Here's the drawing with two shaded views (mm, measured from the low corner). I have some questions. Give positions to 0.01 mm unless a question says otherwise; leave off trailing zeros. Loops run counter-clockwise (first coordinate to the right, second up) from the corner with the lowest first, then second, coordinate; pieces in that order, holes last. Notation, with made-up numbers: (49, 29.25) - (60, 29.25) arc R21 ccw to (60, 53.25) - close; hole circle Ø4 at (-28, 0). An arc over 180 degrees is marked (long way). Use one line per item in the form item = value.
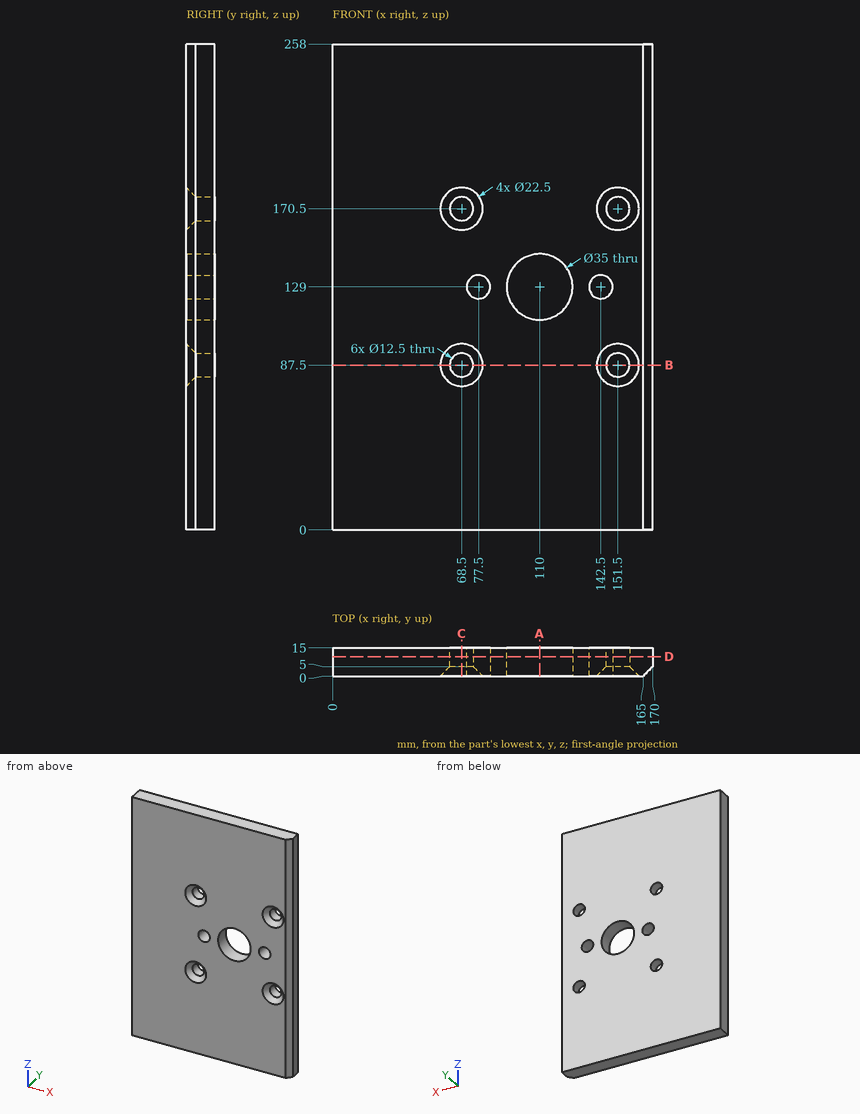
(1) If I drill on probe 1 along Z at (x, y) = (68.5, 11.5); probe 2 along Z at (x, y) = (77.5, 10.25); probe 3 along Z at (x, y) = (149, 3.75), over which ranges is the centre line in solid material (lowest first)?
Geometry says:
probe_1 = 0 to 81.25, 93.75 to 164.25, 176.75 to 258
probe_2 = 0 to 122.75, 135.25 to 258
probe_3 = 0 to 80.43, 94.57 to 163.43, 177.57 to 258
(2) For P1, Ø11, axis at x = 151.5, z = 87.5, coming from the -Y side; P2, Ø16, axis at x = 151.5, z = 170.5, coming from the -Y side; P3, Ø14.5, axis at x = 68.5, z = 170.5, coming from the -Y side, each with a flat end and sliding along its axis, tell me the tip position at first contact or that it passes through.
Geometry says:
P1 = through
P2 = 3.25
P3 = 4
(3) If we section it at C-C (x = 68.5): List the corners of the cut face in (y, z) for me, plus the area to 4 significant figures.
Geometry says:
outline = (0, 0) - (15, 0) - (15, 81.25) - (5, 81.25) - (0, 76.25) - close; (0, 98.75) - (5, 93.75) - (15, 93.75) - (15, 164.25) - (5, 164.25) - (0, 159.25) - close; (0, 181.75) - (5, 176.75) - (15, 176.75) - (15, 258) - (0, 258) - close
area = 3,445 mm²
(4) If we section it at B-B (z = 87.5): List the corners of the cut face in (x, y) for me, plus the area to 3 significant figures.
Geometry says:
outline = (0, 0) - (57.25, 0) - (62.25, 5) - (62.25, 15) - (0, 15) - close; (74.75, 5) - (79.75, 0) - (140.25, 0) - (145.25, 5) - (145.25, 15) - (74.75, 15) - close; (157.75, 5) - (162.75, 0) - (165, 0) - (170, 5) - (170, 15) - (157.75, 15) - close
area = 2,110 mm²
(5) If we section it at D-D (y = 10.25): List the corners of the cut face in (x, z) for me, plus the area to 3 significant figures.
Geometry says:
outline = (0, 0) - (170, 0) - (170, 258) - (0, 258) - close; hole circle Ø12.5 at (68.5, 87.5); hole circle Ø12.5 at (68.5, 170.5); hole circle Ø12.5 at (77.5, 129); hole circle Ø35 at (110, 129); hole circle Ø12.5 at (142.5, 129); hole circle Ø12.5 at (151.5, 87.5); hole circle Ø12.5 at (151.5, 170.5)
area = 42,200 mm²
(6) If we section it at A-A (x = 110): List the corners of the cut face in (y, z) for me.
Geometry says:
outline = (0, 0) - (15, 0) - (15, 111.5) - (0, 111.5) - close; (0, 146.5) - (15, 146.5) - (15, 258) - (0, 258) - close
